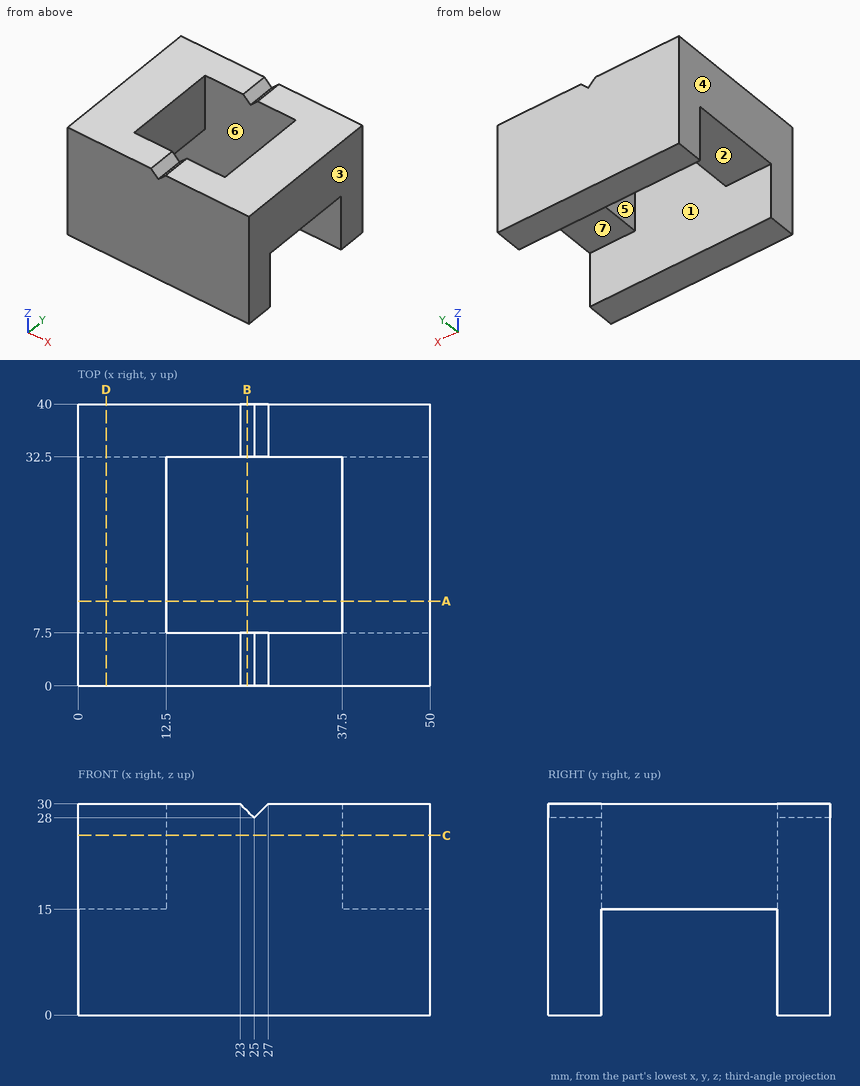
Check sheet for the drawn part. Datum: minimum x, y, z corner. Units: mm. A direction names the side the tool comes from. Coordinates: 2 decimals unless noted, no trailing zeros. Write each loop counter-clockwise with the first axis right and the second up, starting at its lowest first coordinate (ties: lowest second). Pieces come first, ordered by that corner, then holes. Notation, with made-up numbers: (-27, 30) - (18, 30) arc R27 ccw to (18, 65) - close; hole circle Ø2 at (39, 31). An arc over 180 degrees is marked (long way). Answer as a JSON object with one key per item and string values.
(1) Cross-section at C-C on z = 25.5. Record the cut outline in (x, y), plus the area to 4 significant figures.
Report:
{"outline": "(0, 0) - (50, 0) - (50, 40) - (0, 40) - close; hole (12.5, 7.5) - (37.5, 7.5) - (37.5, 32.5) - (12.5, 32.5) - close", "area": "1,375 mm^2"}
(2) Cross-section at A-A on y = 12. Record the cut outline in (x, z).
Report:
{"outline": "(0, 15) - (12.5, 15) - (12.5, 30) - (0, 30) - close; (37.5, 15) - (50, 15) - (50, 30) - (37.5, 30) - close"}
(3) Mould release check, pull along X, two halves, no side actions. Record for the marked faces 1, 2, 3 and 4: pulls with the +X half, pulls with the -X half, needs draft (parallel to the pull), parting line crosses it, or undercut.
Report:
{"face 1": "undercut", "face 2": "needs draft", "face 3": "pulls with the +X half", "face 4": "pulls with the -X half"}
(4) Gauge pin test, flat end, axial feed: pin 1 Ø4 at (x, y) = (5, 20.5) entering from -Z. Record the tip position at first contact, or that the pin passes through.
Report:
{"pin 1": "z = 15"}
(5) Tool access check on the marked faces 5, 6 and 7. Record the directions out of +Z, -Z, +X, -X, +Y, -Y that give a thin tool (end or side, any length) a straight path to the whole face; none if there is none.
Report:
{"face 5": "+Z, -Z", "face 6": "-Z", "face 7": "-Z, +X, -X"}
(6) Cross-section at B-B on x = 24. Record the cut outline in (y, z), plus the area to 3 significant figures.
Report:
{"outline": "(0, 0) - (7.5, 0) - (7.5, 29) - (0, 29) - close; (32.5, 0) - (40, 0) - (40, 29) - (32.5, 29) - close", "area": "435 mm^2"}
(7) Thickness scan on line 1 along Y through (x, z) = (37, 20); line 2 along X through (y, z) = (26, 26.5); line 3 along Z through (x, y) = (3.5, 9.5). Record the ranges inside material, lowest first.
Report:
{"line 1": "0 to 7.5, 32.5 to 40", "line 2": "0 to 12.5, 37.5 to 50", "line 3": "15 to 30"}
(8) Cross-section at D-D on x = 4. Record the cut outline in (y, z), plus the area to 3 significant figures.
Report:
{"outline": "(0, 0) - (7.5, 0) - (7.5, 15) - (32.5, 15) - (32.5, 0) - (40, 0) - (40, 30) - (0, 30) - close", "area": "825 mm^2"}
